Source: CAD feature listing. Evaluate the final solid. Frame: model axes, mm. Face numbers are marked on the shaded views. Coordinates: 2 decimals unless noted, no trailing zeros. Loops run counter-clockwise (first coordinate to the right, second up) from the corner with the lowest first, then second, coordinate; pieces in that order, holes last.
Item 1: Pull-direction query (X, two-part tool) for the marked faces 1 and 2; classes: +X half, -X half, draft (parallel to the pull), parting line (faces both ways), or undercut.
Item 2: Section query C-C, the plane y = -31. Return the cut outline in (x, z), then the cut area to 3 significant figures.
Item 3: Pin query (flat end, axial travel): pin 1 Ø3 at (x, z) = (-35, 5) entering from -Y; pin 2 Ø3 at (x, y) = (-5, 26.5) entering from +Z; pin 3 Ø2 at (y, z) = (20, 1.5) entering from +X; pin 4 Ø1 at (y, z) = (-16.5, 2) entering from -X. Return the tip coordinate at first contact, or that it passes through.
Item 4: Section query B-B, the plane x = -40. Return the cut outline in (y, z).
Item 5: Section query D-D, the plane y = -16.5. Return the cut outline in (x, z).
Item 6: Line query: probe 1 along Y at (x, z) = (-25, 1.45); probe 2 along X at (y, z) = (-46.9, 5); probe 3 along Y at (x, z) = (-19.5, 7.75). Output: solid intervals per line, ascending.
Item 7: Section query A-A, the plane x = 16. Return the cut outline in (y, z).
```python
from build123d import *

# Parameters (mm, degrees)
SKETCH1_W                      = 96
SKETCH1_H                      = 96
BOSS_EXTRUDE1_DEPTH            = 8
SKETCH2_W                      = 92
SKETCH2_H                      = 92
COMPONENT_PLATFORM_DEPTH       = 6
CABLE_SLOTS_DEPTH              = 6
INNER_CORNER_FILLETS_R         = 3
M3X0_5_TAPPED_HOLE1_AT_2_COUNT = 2
M3X0_5_TAPPED_HOLE1_AT_2_PITCH = 70
M3X0_5_TAPPED_HOLE2_AT_2_COUNT = 2
M3X0_5_TAPPED_HOLE2_AT_2_PITCH = 70
SKETCH29_R                     = 12
HDD_EXTRUSION_CUTOUT_DEPTH     = 10
HDD_EXTRUSION_CUTOUT_2_DEPTH   = 10
F_3_0MM_DOWEL_HOLE1_D          = 3
F_3_0MM_DOWEL_HOLE1_DEPTH      = 2
F_3_0MM_DOWEL_HOLE2_D          = 3
CUT_EXTRUDE1_START             = -8
SKETCH35_OUTSIDE_W             = 125.2
SKETCH35_OUTSIDE_H             = 125.2
SKETCH35_OUTSIDE_W_2           = 95
SKETCH35_OUTSIDE_H_2           = 95
CUT_EXTRUDE1_DEPTH             = 8
M1_6_CLEARANCE_HOLE2_D         = 1


with BuildPart() as part:
    # Sketch1 → Boss-Extrude1 (new body)
    with BuildSketch(Plane.XY):
        Rectangle(SKETCH1_W, SKETCH1_H)
    extrude(amount=BOSS_EXTRUDE1_DEPTH)

    # Sketch2 → Component Platform (cut)
    with BuildSketch(Plane.XY.offset(8)):
        Rectangle(SKETCH2_W, SKETCH2_H)
    extrude(amount=-COMPONENT_PLATFORM_DEPTH, mode=Mode.SUBTRACT)

    # Sketch3 → Cable Slots (cut, symmetric)
    with BuildSketch(Plane.XY.offset(2)):
        with BuildLine():
            Line((-33.878679656, -25.121320344), (-28.878679656, -20.121320344))
            ThreePointArc((-28.878679656, -20.121320344), (-28.228361402, -19.148050297), (-28, -18))
            Line((-28, -18), (-28, 18))
            ThreePointArc((-28, 18), (-28.228361402, 19.148050297), (-28.878679656, 20.121320344))
            Line((-28.878679656, 20.121320344), (-33.878679656, 25.121320344))
            ThreePointArc((-33.878679656, 25.121320344), (-34.851949703, 25.771638598), (-36, 26))
            Line((-36, 26), (-48, 26))
            Line((-48, 26), (-48, -26))
            Line((-48, -26), (-36, -26))
            ThreePointArc((-36, -26), (-34.851949703, -25.771638598), (-33.878679656, -25.121320344))
        make_face()
        with BuildLine():
            Line((48, -26), (48, 26))
            Line((48, 26), (36, 26))
            ThreePointArc((36, 26), (34.851949703, 25.771638598), (33.878679656, 25.121320344))
            Line((33.878679656, 25.121320344), (28.878679656, 20.121320344))
            ThreePointArc((28.878679656, 20.121320344), (28.228361402, 19.148050297), (28, 18))
            Line((28, 18), (28, -18))
            ThreePointArc((28, -18), (28.228361402, -19.148050297), (28.878679656, -20.121320344))
            Line((28.878679656, -20.121320344), (33.878679656, -25.121320344))
            ThreePointArc((33.878679656, -25.121320344), (34.851949703, -25.771638598), (36, -26))
            Line((36, -26), (48, -26))
        make_face()
    extrude(amount=CABLE_SLOTS_DEPTH, both=True, mode=Mode.SUBTRACT)

    # Inner Corner Fillets
    inner_corner_fillets_edges = [part.edges().sort_by_distance(p)[0] for p in [
        (-46, -46, 5),
        (-46, 46, 5),
        (46, 46, 5),
        (46, -46, 5),
    ]]
    fillet(inner_corner_fillets_edges, radius=INNER_CORNER_FILLETS_R)

    # Sketch14 → M3x0.5 Tapped Hole1 (revolve, cut)
    with BuildSketch(Plane(origin=(48, -35, 5), x_dir=(0, 0, -1), z_dir=(0, 1, 0))):
        Polygon((0, 0), (0, 10.751075774), (1.25, 10), (1.25, 0), align=None)
    m3x0_5_tapped_hole1 = revolve(axis=Axis((54.35, -35, 5), (-1, 0, 0)), mode=Mode.SUBTRACT)

    # M3x0.5 Tapped Hole1 at 2: M3x0.5 Tapped Hole1 ×2
    with Locations(*[(0, i * M3X0_5_TAPPED_HOLE1_AT_2_PITCH, 0) for i in range(1, M3X0_5_TAPPED_HOLE1_AT_2_COUNT)]):
        add(m3x0_5_tapped_hole1, mode=Mode.SUBTRACT)

    # Sketch16 → M3x0.5 Tapped Hole2 (revolve, cut)
    with BuildSketch(Plane(origin=(35, 48, 5), x_dir=(0, 0, 1), z_dir=(1, 0, 0))):
        Polygon((0, 0), (0, 10.751075774), (1.25, 10), (1.25, 0), align=None)
    m3x0_5_tapped_hole2 = revolve(axis=Axis((35, 54.35, 5), (0, -1, 0)), mode=Mode.SUBTRACT)

    # M3x0.5 Tapped Hole2 at 2: M3x0.5 Tapped Hole2 ×2
    with Locations(*[(-i * M3X0_5_TAPPED_HOLE2_AT_2_PITCH, 0, 0) for i in range(1, M3X0_5_TAPPED_HOLE2_AT_2_COUNT)]):
        add(m3x0_5_tapped_hole2, mode=Mode.SUBTRACT)

    # Mirror1: M3x0.5 Tapped Hole1 across plane
    add(m3x0_5_tapped_hole1.mirror(Plane(origin=(0, 0, 0), x_dir=(0, 0, 1), z_dir=(1, 0, 0))), mode=Mode.SUBTRACT)

    # Mirror1 copy 1 sketch → Mirror1 copy 1 (revolve, cut)
    with BuildSketch(Plane(origin=(-48, 35, 5), x_dir=(0, 0, -1), z_dir=(0, 1, 0))):
        Polygon((0, 0), (0, -10.751075774), (1.25, -10), (1.25, 0), align=None)
    revolve(axis=Axis((-54.35, 35, 5), (-1, 0, 0)), mode=Mode.SUBTRACT)

    # Mirror2: M3x0.5 Tapped Hole2 across plane
    add(m3x0_5_tapped_hole2.mirror(Plane(origin=(0, 0, 0), x_dir=(0, 0, 1), z_dir=(0, -1, 0))), mode=Mode.SUBTRACT)

    # Mirror2 copy 1 sketch → Mirror2 copy 1 (revolve, cut)
    with BuildSketch(Plane(origin=(-35, -48, 5), x_dir=(0, 0, 1), z_dir=(1, 0, 0))):
        Polygon((0, 0), (0, -10.751075774), (1.25, -10), (1.25, 0), align=None)
    revolve(axis=Axis((-35, -54.35, 5), (0, -1, 0)), mode=Mode.SUBTRACT)

    # Sketch29 → HDD Extrusion Cutout (cut)
    with BuildSketch(Plane(origin=(0, 0, 0), x_dir=(-1, 0, 0), z_dir=(0, 0, -1))):
        with Locations((-0.08192631, -8.74785827)):
            Circle(SKETCH29_R)
    extrude(amount=-HDD_EXTRUSION_CUTOUT_DEPTH, mode=Mode.SUBTRACT)

    # Sketch9 → HDD Extrusion Cutout 2 (cut)
    with BuildSketch(Plane.XY.offset(2)):
        with BuildLine():
            Line((24.5, 31), (24.5, 9))
            ThreePointArc((24.5, 9), (23.914213562, 7.585786438), (22.5, 7))
            Line((22.5, 7), (14.5, 7))
            ThreePointArc((14.5, 7), (13.085786438, 7.585786438), (12.5, 9))
            Line((12.5, 9), (12.5, 10))
            ThreePointArc((12.5, 10), (11.914213562, 11.414213562), (10.5, 12))
            Line((10.5, 12), (-6, 12))
            ThreePointArc((-6, 12), (-7.414213562, 12.585786438), (-8, 14))
            Line((-8, 14), (-8, 31))
            ThreePointArc((-8, 31), (-7.414213562, 32.414213562), (-6, 33))
            Line((-6, 33), (22.5, 33))
            ThreePointArc((22.5, 33), (23.914213562, 32.414213562), (24.5, 31))
        make_face()
    extrude(amount=-HDD_EXTRUSION_CUTOUT_2_DEPTH, mode=Mode.SUBTRACT)

    # Ø3.0mm Dowel Hole1
    with Locations(Plane.XY.offset(2)):
        with Locations((-31.790998517, -39.06), (31.29001483, -39.06), (31.29001483, 38.94), (-31.790998517, 38.94)):
            Hole(F_3_0MM_DOWEL_HOLE1_D / 2, depth=F_3_0MM_DOWEL_HOLE1_DEPTH)

    # Ø3.0mm Dowel Hole2 (through all)
    with Locations(Plane.XY.offset(2)):
        with Locations((40, -40), (-40, -40), (-40, 40), (40, 40)):
            Hole(F_3_0MM_DOWEL_HOLE2_D / 2)

    # Sketch35 outside → Cut-Extrude1 (cut)
    with BuildSketch(Plane(origin=(0, 0, 0), x_dir=(-1, 0, 0), z_dir=(0, 0, -1)).offset(CUT_EXTRUDE1_START)):
        Rectangle(SKETCH35_OUTSIDE_W, SKETCH35_OUTSIDE_H)
        Rectangle(SKETCH35_OUTSIDE_W_2, SKETCH35_OUTSIDE_H_2, mode=Mode.SUBTRACT)
    extrude(amount=CUT_EXTRUDE1_DEPTH, mode=Mode.SUBTRACT)

    # M1.6 Clearance Hole2 (through all)
    with Locations(Plane(origin=(-25, -33.5, 2), x_dir=(1, 0, 0), z_dir=(0, 0, 1))):
        with Locations((0, 0), (0, 36.6), (1.6, 41.7), (0, 67), (50, 67), (50, 36.6)):
            Hole(M1_6_CLEARANCE_HOLE2_D / 2)


solid = part.part
```
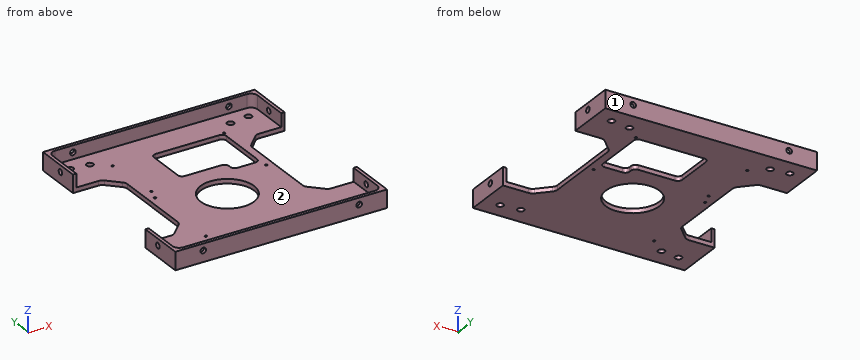
Verdict:
1. face 1: draft
1. face 2: undercut
2. outline: (-47.5, 0) - (47.5, 0) - (47.5, 8) - (46, 8) - (46, 2) - (-46, 2) - (-46, 8) - (-47.5, 8) - close
2. area: 208 mm2
3. pin 1: stops at y = -47.5
3. pin 2: passes through
3. pin 3: stops at x = 29.76
3. pin 4: stops at x = -28
4. outline: (-47.5, 0) - (-41.5, 0) - (-41.5, 2) - (-46, 2) - (-46, 8) - (-47.5, 8) - close; (-38.5, 0) - (-26, 0) - (-26, 2) - (-38.5, 2) - close; (26, 0) - (38.5, 0) - (38.5, 2) - (26, 2) - close; (41.5, 0) - (47.5, 0) - (47.5, 8) - (46, 8) - (46, 2) - (41.5, 2) - close
5. outline: (-28, 0) - (-9.08, 0) - (-9.08, 2) - (-28, 2) - close; (9.24, 0) - (28, 0) - (28, 2) - (9.24, 2) - close
6. probe 1: y = -47.5 to -34, -33 to 2.6, 3.6 to 33, 34 to 47.5
6. probe 2: x = -47.5 to -36.25, -33.75 to 33.75, 36.25 to 47.5
6. probe 3: y = -47.5 to -46, 46 to 47.5
7. outline: (-47.5, 0) - (7, 0) - (7, 2) - (-46, 2) - (-46, 8) - (-47.5, 8) - close; (33, 0) - (47.5, 0) - (47.5, 8) - (46, 8) - (46, 2) - (33, 2) - close
